Geometry: final body of the model. Coordinates: model frame, mm. A direction names the side the tool comes from. Round coordinates to 2 decimals unless told otherwise and drop trailing zeros. Loops run counter-clockwise (first coordinate to the right, second up) from the corner with the lowest first, then second, coordinate; pieces in that order, holes last. Notation, with made-up numbers: M -28.75,79 L -19.75,79 A25 cw -19.75,109 Z; hole C 8,33.5 d6. An arc over 180 degrees is marked long. Answer as a JSON object with one key per item and string values.
from build123d import *

# Parameters (mm, degrees)
F2_R     = 1.28
F3_DEPTH = 34.659312
F4_R     = 2
F5_R     = 2


with BuildPart() as f1:
    # F0 (on Front) → F1 (revolve)
    with BuildSketch(Plane.XZ):
        Polygon((-15, 0), (0, 0), (0, 34.658312), (-5, 34.658312), (-7.5, 33), (-7.5, 27), (-21.5, 27), (-21.5, 15), (-15, 15), align=None)
    revolve(axis=Axis((0, 0, 25.863634), (0, 0, 1)))

    # F2 (on face) → F3 (cut, through all)
    with BuildSketch(Plane.XY.offset(34.658312)):
        Circle(F2_R)
    extrude(amount=-F3_DEPTH, mode=Mode.SUBTRACT)

    # F4
    f4_edges = [f1.edges().sort_by_distance(p)[0] for p in [
        (21.5, 0, 15),
    ]]
    fillet(f4_edges, radius=F4_R)

    # F5
    f5_edges = [f1.edges().sort_by_distance(p)[0] for p in [
        (15, 0, 0),
    ]]
    fillet(f5_edges, radius=F5_R)


solid = f1.part
1) Section query C-C (z = 5). Return the cut outline in (x, y).
Results:
{"outline": "C 0,0 d30; hole C 0,0 d2.56"}
2) Reachability of faces 1 (the cylindrical face through (2.799, -21.317, 21.93)), 2 (the flat face through (-10, 11.5, 15)), 3 (the flat face through (9, 0, 27)) from +Z, -Z, +X, -X, +Y, -Y: full face, straight path, thin tool, end or side. Return the list, or none.
Results:
{"face 1": "+Z, -Z", "face 2": "-Z", "face 3": "+Z"}
3) Pull-direction query (Y, two-part tool) for faces 4 (the cylindrical face through (-1.28, 0.06, 17.57)), 5 (the cylindrical face through (7.493, -0.33, 29.958)), 6 (the flat face through (-3, 0, 0)); classes: +Y half, -Y half, draft (parallel to the pull), parting line (faces both ways), or undercut.
Results:
{"face 4": "undercut", "face 5": "parting line", "face 6": "draft"}
4) Ray query, line 1 (Y direction, x = 0, z = 14); line 2 (Y direction, x = 0, z = 22); line 3 (Z direction, x = -10, y = -3). Return the intervals inside material, ascending.
Results:
{"line 1": "-15 to -1.28, 1.28 to 15", "line 2": "-21.5 to -1.28, 1.28 to 21.5", "line 3": "0 to 27"}
5) Section query A-A (x = 0). Return the cut outline in (y, z), and give its area (3 significant figures).
Results:
{"outline": "M -21.5,17 A2 ccw -19.5,15 L -15,15 L -15,2 A2 ccw -13,0 L -1.28,0 L -1.28,34.66 L -5,34.66 L -7.5,33 L -7.5,27 L -21.5,27 Z; M 1.28,0 L 13,0 A2 ccw 15,2 L 15,15 L 19.5,15 A2 ccw 21.5,17 L 21.5,27 L 7.5,27 L 7.5,33 L 5,34.66 L 1.28,34.66 Z", "area": "985 mm2"}
6) Pin query (flat end, axial travel): P1, Ø5, axis at x = 1.5, z = 3.5, coming from the +Y side; P2, Ø2, axis at y = -3, z = 15, coming from the +X side; P3, Ø1.5, axis at x = 11.5, y = -1.5, coming from the -Z side; P4, Ø2, axis at x = -16.5, y = 10, coming from the +Z side. Return the tip coordinate at first contact, or that it passes through.
Results:
{"P1": "y = 15", "P2": "x = 21.03", "P3": "z = 0", "P4": "z = 27"}
